from build123d import *

# Parameters (mm, degrees)
PAD_DEPTH    = 32
PAD001_DEPTH = 15
SKETCH002_R  = 10
POCKET_DEPTH = 15.001


with BuildPart() as part:
    # Sketch → Pad (new body, symmetric)
    with BuildSketch(Plane.XZ):
        with BuildLine():
            ThreePointArc((25, 0), (0, 25), (-25, 0))
            Line((-40, 0), (-25, 0))
            ThreePointArc((40, 0), (0, 40), (-40, 0))
            Line((25, 0), (40, 0))
        make_face()
    extrude(amount=PAD_DEPTH, both=True)

    # Sketch001 → Pad001 (join)
    with BuildSketch(Plane.XY):
        with BuildLine():
            Line((65, 25), (25, 25))
            Line((25, 25), (25, -25))
            Line((25, -25), (65, -25))
            ThreePointArc((65, -25), (90, 0), (65, 25))
        make_face()
    extrude(amount=PAD001_DEPTH)

    # Sketch002 (on Face10 of Pad001) → Pocket (cut, through all)
    with BuildSketch(Plane(origin=(0, 0, 15), x_dir=(-1, 0, 0), z_dir=(0, 0, 1))):
        with Locations((-65, 0)):
            Circle(SKETCH002_R)
    extrude(amount=-POCKET_DEPTH, mode=Mode.SUBTRACT)


solid = part.part
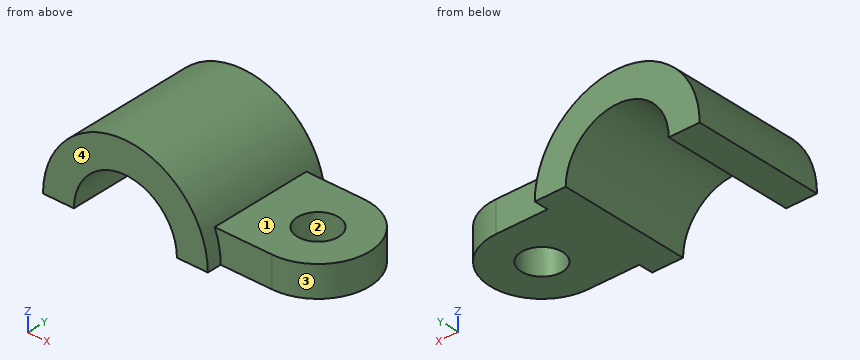
Here's how the part is built. I have some questions about the finished solid (model axes, mm). Face numbers are marked on the shaded views. Give positions to 0.01 mm unless a question says otherwise; leave off trailing zeros. Loops run counter-clockwise (first coordinate to the right, second up) from the corner with the lowest first, then second, coordinate; pieces in that order, holes last. Notation, with made-up numbers: (88.5, -39) -> (102.5, -39) arc R12 ccw to (102.5, -24) -> close; hole circle Ø4 at (62, 40). An arc over 180 degrees is marked (long way). Answer as a JSON object with one key per item and string values. Group by question number.
Item 1: Will these pins go through, and if not, where does the flat tip stop? pin 1 (4 mm diameter, centred on y = -14.5, z = 12, fed in from -X); pin 2 (1 mm diameter, centred on y = -24.5, z = 12.5, fed in from -X); pin 3 (5 mm diameter, centred on y = 15.5, z = 24, fed in from +X).
Item 2: Imagine slicing it at D-D on y = 22. Write out the boundary of the cut face in (x, z), then the cut area to 3 significant figures.
Item 3: Imagine slicing it at C-C on x = 62. Write out the boundary of the cut face in (y, z), then the cut area to 3 significant figures.
Item 4: Imagine slicing it at A-A on z = 8.5. Write out the boundary of the cut face in (x, y), then the cut area to 3 significant figures.
Item 5: Imagine slicing it at B-B on y = 0. Write out the boundary of the cut face in (x, z), then the cut area to 3 significant figures.
Item 6: Thinking about a two-plate mould opening in Y: for the marked faces 1, 2, 3 and 4, which applies, pulls with the +Y half, pulls with the -Y half, needs draft (parallel to the pull), parting line crosses it, or undercut?
Item 7: I need wall thicknesses on L1, parallel to Y at x = 65, z = 7; L2, parallel to X at y = 0, z = 4; L3, parallel to X at y = 0, z = 11.25. Which ranges of each line are inside material? Lowest first, please.
Answer list:
{
 "1": {"pin 1": "stops at x = -38.73", "pin 2": "stops at x = -38.16", "pin 3": "stops at x = 33.73"},
 "2": {"outline": "(-40, 0) -> (-25, 0) arc R25 cw to (25, 0) -> (76.87, 0) -> (76.87, 15) -> (37.08, 15) arc R40 ccw to start", "area": "2,100 mm2"},
 "3": {"outline": "(-25, 0) -> (-9.54, 0) -> (-9.54, 15) -> (-25, 15) -> close; (9.54, 0) -> (25, 0) -> (25, 15) -> (9.54, 15) -> close", "area": "464 mm2"},
 "4": {"outline": "(-39.09, -32) -> (-23.51, -32) -> (-23.51, 32) -> (-39.09, 32) -> close; (23.51, -32) -> (39.09, -32) -> (39.09, -25) -> (65, -25) arc R25 ccw to (65, 25) -> (39.09, 25) -> (39.09, 32) -> (23.51, 32) -> close; hole circle Ø20 at (65, 0)", "area": "3,960 mm2"},
 "5": {"outline": "(-40, 0) -> (-25, 0) arc R25 cw to (25, 0) -> (55, 0) -> (55, 15) -> (37.08, 15) arc R40 ccw to start; (75, 0) -> (90, 0) -> (90, 15) -> (75, 15) -> close", "area": "2,000 mm2"},
 "6": {"face 1": "needs draft", "face 2": "undercut", "face 3": "parting line crosses it", "face 4": "pulls with the -Y half"},
 "7": {"L1": "y = -25 to -10, 10 to 25", "L2": "x = -39.8 to -24.68, 24.68 to 55, 75 to 90", "L3": "x = -38.39 to -22.33, 22.33 to 55, 75 to 90"}
}
